Geometry check sheet. Reference: the model listing, model coordinates, mm. A direction names the side the tool comes from. Round coordinates to 2 decimals unless told otherwise and drop trailing zeros. Order: outer loops, then holes, each group sorted by start corner. A loop starts at its lowest first (then second) coordinate and runs counter-clockwise, first axis right, second up. Notation, with made-up numbers: (47, 27) -> (100, 27) arc R11 cw to (100, 42) -> close; hole circle Ø8 at (-23.5, 49). An arc over 180 degrees is marked (long way). Use a Markdown table: item, result. Add a question column.
Item 1: Material ranges on probe 1 along Y at (x, z) = (-24.5, 28); probe 2 along X at (y, z) = (32.5, 20); probe 3 along Y at (x, z) = (0, 18), recorded low to high. Write a range as [from, to].
Item 2: Gauge pin test, flat ends, axial feed: pin 1 Ø8 at (y, z) = (-2, 7.5) entering from +X; pin 2 Ø10 at (y, z) = (16, 21) entering from +X; pin 3 Ø2 at (y, z) = (-3.5, 38) entering from +X; pin 4 Ø8 at (y, z) = (10, 12) entering from -X. Record the tip position at first contact, or that the pin passes through.
Item 3: Mould release check, pull along Y, two halves, no side actions. Record for faces 1 (the cylindrical face through (-29.04, 41.19, 24.65)), 2 (the cylindrical face through (12.539, 20.492, 25.35)), 3 (the flat face through (-8, 14, 50)), 4 (the flat face through (33.22, -25.68, 24.65)): pulls with the +Y half, pulls with the -Y half, needs draft (parallel to the pull), parting line crosses it, or undercut.
Item 4: Set-up check for faces 5 (the flat face through (17.232, 25.717, 25.35)), 6 (the flat face through (-45, -26, 50)), 7 (the cylindrical face through (29.27, 30.54, 2.46)), 8 (the flat face through (28.635, 44.191, 2.535)), 9 (the flat face through (-43, -19, 45)): record each of +Z, -Z, +X, -X, +Y, -Y from which the full face is reachable in a straight line by a thin tool's end or side.
Item 5: Sectioned sample at B-B, the plane y = 0. State how many separate pieces and enclosed holes the cut face has, and give its area (3 significant figures).
Item 6: Sectioned sample at A-A, the plane x = 0. Record the cut outline in (y, z), and give its area (3 significant figures).
from build123d import *

# Parameters (mm, degrees)
SKETCH1_R           = 11
BOSS_EXTRUDE1_DEPTH = 50
FILLET2_R           = 25
FILLET5_R           = 5
CUT_EXTRUDE2_DEPTH  = 50
FILLET6_R           = 3.5
CUT_EXTRUDE3_DEPTH  = 5
CUT_EXTRUDE4_START  = -45
CUT_EXTRUDE4_DEPTH  = 5
CUT_EXTRUDE1_DEPTH  = 20
FILLET8_R           = 3


with BuildPart() as part:
    # Sketch1 → Boss-Extrude1 (new body)
    with BuildSketch(Plane.XY):
        with BuildLine():
            Line((-47.101242547, -32.98064509), (-15.03971276, -10.530920247))
            ThreePointArc((-15.03971276, -10.530920247), (-11.176920202, -14.566045997), (-6.279523746, -17.252849698))
            Line((-6.279523746, -17.252849698), (31.308181085, -30.933655431))
            Line((31.308181085, -30.933655431), (43.278886102, 1.955586297))
            Line((43.278886102, 1.955586297), (12.982550619, 12.982550619))
            Line((12.982550619, 12.982550619), (40.658639918, 40.658639918))
            ThreePointArc((40.658639918, 40.658639918), (-36.960287557, 44.047555479), (-47.101242547, -32.98064509))
        make_face()
        Circle(SKETCH1_R, mode=Mode.SUBTRACT)
    extrude(amount=BOSS_EXTRUDE1_DEPTH)

    # Fillet2
    fillet2_edges = [part.edges().sort_by_distance(p)[0] for p in [
        (-15.03971276, -10.530920247, 25),
    ]]
    fillet(fillet2_edges, radius=FILLET2_R)

    # Fillet5
    fillet5_edges = [part.edges().sort_by_distance(p)[0] for p in [
        (12.982550619, 12.982550619, 25),
    ]]
    fillet(fillet5_edges, radius=FILLET5_R)

    # Sketch4 → Cut-Extrude2 (cut)
    with BuildSketch(Plane.XY.offset(50)):
        with BuildLine():
            Line((-42.148022243, -6.317645709), (-34.691528571, -16.966622285))
            Line((-34.691528571, -16.966622285), (-32.46214687, -15.405592412))
            ThreePointArc((-32.46214687, -15.405592412), (-23.62229066, -11.116679876), (-13.884259621, -9.809553241))
            ThreePointArc((-13.884259621, -9.809553241), (-16.986342471, 0.681299827), (-13.054027301, 10.890012453))
            Line((-13.054027301, 10.890012453), (-35.345481592, 37.455933189))
            ThreePointArc((-35.345481592, 37.455933189), (-49.339432978, 14.76043202), (-50.108305856, -11.891496301))
            Line((-50.108305856, -11.891496301), (-42.148022243, -6.317645709))
        make_face()
        with BuildLine():
            ThreePointArc((20.41205375, 47.282111435), (-5.968485267, 51.152978248), (-30.749214933, 41.312658847))
            Line((-30.749214933, 41.312658847), (-8.457760642, 14.746738111))
            ThreePointArc((-8.457760642, 14.746738111), (1.75926732, 16.908724922), (11.312388901, 12.68975403))
            ThreePointArc((11.312388901, 12.68975403), (11.517857333, 18.111100205), (14.289586512, 22.774867886))
            Line((14.289586512, 22.774867886), (22.732981885, 31.218263259))
            Line((22.732981885, 31.218263259), (13.54059373, 40.410651415))
            Line((13.54059373, 40.410651415), (20.41205375, 47.282111435))
        make_face()
    extrude(amount=-CUT_EXTRUDE2_DEPTH, mode=Mode.SUBTRACT)

    # Fillet6
    fillet6_edges = [part.edges().sort_by_distance(p)[0] for p in [
        (-13.884259621, -9.809553241, 25),
        (-13.054027301, 10.890012453, 25),
        (-35.345481592, 37.455933189, 25),
        (-30.749214933, 41.312658847, 25),
        (-8.457760642, 14.746738111, 25),
        (11.312388901, 12.68975403, 25),
        (-50.108305856, -11.891496301, 25),
        (-34.691528571, -16.966622285, 25),
        (-42.148022243, -6.317645709, 25),
        (22.732981885, 31.218263259, 25),
        (13.54059373, 40.410651415, 25),
        (20.41205375, 47.282111435, 25),
    ]]
    fillet(fillet6_edges, radius=FILLET6_R)

    # Sketch4<3> → Cut-Extrude3 (cut)
    with BuildSketch(Plane.XY.offset(50)):
        with BuildLine():
            Line((-52.540659522, -23.360845383), (-47.522133036, -19.846835307))
            ThreePointArc((-47.522133036, -19.846835307), (-48.096606551, -18.411041206), (-48.627711525, -16.958645933))
            Line((-48.627711525, -16.958645933), (-53.713864559, -20.520008628))
            ThreePointArc((-53.713864559, -20.520008628), (-53.146246907, -21.948267351), (-52.540659522, -23.360845383))
        make_face()
        with BuildLine():
            Line((-44.112627107, -17.459473554), (-41.244744925, -21.555233775))
            Line((-41.244744925, -21.555233775), (-38.787288792, -19.834504466))
            Line((-38.787288792, -19.834504466), (-43.375900283, -13.281288112))
            Line((-43.375900283, -13.281288112), (-48.627711525, -16.958645933))
            ThreePointArc((-48.627711525, -16.958645933), (-48.096606551, -18.411041206), (-47.522133036, -19.846835307))
            Line((-47.522133036, -19.846835307), (-44.112627107, -17.459473554))
        make_face()
        Polygon((-38.787288792, -19.834504466), (-41.244744925, -21.555233775), (-37.803286307, -26.470146041), (-35.345830174, -24.749416732), align=None)
    extrude(amount=-CUT_EXTRUDE3_DEPTH, mode=Mode.SUBTRACT)

    # Sketch4<4> → Cut-Extrude4 (cut)
    with BuildSketch(Plane.XY.offset(50).offset(CUT_EXTRUDE4_START)):
        with BuildLine():
            ThreePointArc((32.12953143, 47.685880616), (30.843572778, 48.527559369), (29.535578285, 49.334568158))
            Line((29.535578285, 49.334568158), (25.145119486, 44.944109359))
            ThreePointArc((25.145119486, 44.944109359), (26.4832242, 44.168867271), (27.797449084, 43.35379827))
            Line((27.797449084, 43.35379827), (32.12953143, 47.685880616))
        make_face()
        with BuildLine():
            ThreePointArc((27.797449084, 43.35379827), (26.4832242, 44.168867271), (25.145119486, 44.944109359))
            Line((25.145119486, 44.944109359), (20.611661542, 40.410651415))
            Line((20.611661542, 40.410651415), (26.268515791, 34.753797165))
            Line((26.268515791, 34.753797165), (28.389836135, 36.875117509))
            Line((28.389836135, 36.875117509), (24.854302229, 40.410651415))
            Line((24.854302229, 40.410651415), (27.797449084, 43.35379827))
        make_face()
        Polygon((28.389836135, 36.875117509), (26.268515791, 34.753797165), (30.511156478, 30.511156478), (32.632476822, 32.632476822), align=None)
    extrude(amount=-CUT_EXTRUDE4_DEPTH, mode=Mode.SUBTRACT)

    # Sketch2 → Cut-Extrude1 (cut)
    with BuildSketch(Plane(origin=(37.587704831, -13.680805733, 0), x_dir=(0, 0, -1), z_dir=(0.939692620785907, -0.34202014332567265, 0))):
        with BuildLine():
            ThreePointArc((-13.5, -0.86009916), (-21.542647074, 10.107886559), (-34.421167086, 5.7347178))
            Line((-34.421167086, 5.7347178), (-15.578832914, -7.45491612))
            ThreePointArc((-15.578832914, -7.45491612), (-14.03201428, -4.317452086), (-13.5, -0.86009916))
        make_face()
        with BuildLine():
            Line((-15.578832914, -7.45491612), (-34.421167086, 5.7347178))
            ThreePointArc((-34.421167086, 5.7347178), (-31.59481696, -10.281266246), (-15.578832914, -7.45491612))
        make_face()
    extrude(amount=-CUT_EXTRUDE1_DEPTH, mode=Mode.SUBTRACT)

    # Fillet8
    fillet8_edges = [part.edges().sort_by_distance(p)[0] for p in [
        (-44.112627107, -17.459473554, 47.5),
        (-52.540659522, -23.360845383, 47.5),
        (-53.713864559, -20.520008628, 47.5),
        (-43.375900283, -13.281288112, 47.5),
        (-35.345830174, -24.749416732, 47.5),
        (-37.803286307, -26.470146041, 47.5),
        (30.511156478, 30.511156478, 2.5),
        (32.632476822, 32.632476822, 2.5),
        (24.854302229, 40.410651415, 2.5),
        (32.12953143, 47.685880616, 2.5),
        (29.535578285, 49.334568158, 2.5),
        (20.611661542, 40.410651415, 2.5),
    ]]
    fillet(fillet8_edges, radius=FILLET8_R)


solid = part.part
Found:
| question | item | result |
|---|---|---|
| 1 | probe 1 | y = [-17.81, -11.4], [24.53, 33.87], [45.3, 52.02] |
| 1 | probe 2 | x = [-47.43, -39.95], [-31.19, -23.35], [21.04, 32.5] |
| 1 | probe 3 | y = [-19.54, -11], [11, 17], [51.5, 57.5] |
| 2 | pin 1 | stops at x = 43.28 |
| 2 | pin 2 | stops at x = 21 |
| 2 | pin 3 | stops at x = 41.66 |
| 2 | pin 4 | stops at x = -57.19 |
| 3 | face 1 | undercut |
| 3 | face 2 | undercut |
| 3 | face 3 | needs draft |
| 3 | face 4 | pulls with the -Y half |
| 4 | face 5 | +Z, -Z |
| 4 | face 6 | +Z, +X, -X, +Y, -Y |
| 4 | face 7 | -Z, +X |
| 4 | face 8 | -Z |
| 4 | face 9 | +Z |
| 5 | separate pieces | 3 |
| 5 | enclosed holes | 1 |
| 5 | area | 2,070 mm2 |
| 6 | outline | (-19.54, 0) -> (-11, 0) -> (-11, 50) -> (-19.54, 50) -> close; (11, 0) -> (17, 0) -> (17, 50) -> (11, 50) -> close; (51.5, 0) -> (57.5, 0) -> (57.5, 50) -> (51.5, 50) -> close |
| 6 | area | 1,030 mm2 |
